The listing builds one solid part. Answer for the finished solid, in the listing's coordinates (mm). Face numbers are marked on the shaded views. A direction names the side the tool comes from. Give positions to 0.01 mm unless a question says otherwise; leave off trailing zeros. Loops run counter-clockwise (first coordinate to the right, second up) from the corner with the lowest first, then second, coordinate; pieces in that order, holes last. Notation, with made-up numbers: M -32,-33.5 L 12,-33.5 A32 cw 12,5.5 Z; hole C 39.5,84 d5. An arc over 180 degrees is marked long. One line per item, written item: value. Start each with the question number.
Q1. A cutting plane is placed at A-A, the plane x = 0. Determine the outline of the cut face in (y, z) (3 decimals), and give its area (3 significant figures).
Q2. The mould has two halves that part along Y. Classify the marked faces 1, 2 and 3: +Y half, -Y half, draft (parallel to the pull), parting line (faces both ways), or undercut.
Q3. A cutting plane is placed at C-C, the plane z = -1. Determine the outline of the cut face in (x, y) (3 decimals).
Q4. A cutting plane is placed at D-D, the plane z = 2.25. Determine the outline of the cut face in (x, y), and give its area (3 significant figures).
Q5. Flat-ended cylindrical pins translate along their axes: pin 1 (12 mm diameter, centred on x = 0, y = 0, fed in from +Z); pin 2 (1 mm diameter, centred on y = 6.5, z = -1, fed in from -X); pin 3 (4 mm diameter, centred on x = 5.5, z = 0.5, fed in from -Y). Find the tip coordinate at first contact, or state that the pin passes through.
Q6. For the marked faces 4 and 5, determine the directions among +Z, -Z, +X, -X, +Y, -Y from which every point of the face is accessible in a straight line to the end or side of a thin tool.
Q7. Consider L1, parallel to Y at x = 0, z = 1.8; L2, parallel to Z at x = 3, y = 0.25. Determine where each line is inside the solid, lowest interval first.
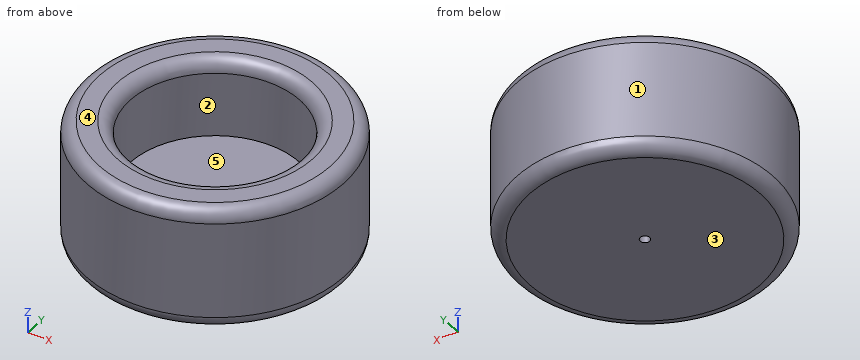
from build123d import *

# Parameters (mm, degrees)
F0_R     = 10
F1_DEPTH = 3.5
F2_R     = 10
F2_R_2   = 6.6
F3_DEPTH = 6
F4_R     = 1
F5_R     = 1
F6_R     = 0.375
F7_DEPTH = 3.501


# Not quite as in the source:
# - a feature names something its author has since deleted; it is built from what else it names


with BuildPart() as f1:
    # F0 (on Top) → F1 (new body)
    with BuildSketch(Plane.XY):
        Circle(F0_R)
    extrude(amount=-F1_DEPTH)

    # F2 (on face) → F3 (join)
    with BuildSketch(Plane.XY):
        Circle(F2_R)
        Circle(F2_R_2, mode=Mode.SUBTRACT)
    extrude(amount=F3_DEPTH)

    # F4
    f4_edges = [f1.edges().sort_by_distance(p)[0] for p in [
        (-6.6, 0, 6),
        (-10, 0, -3.5),
    ]]
    fillet(f4_edges, radius=F4_R)

    # F5
    f5_edges = [f1.edges().sort_by_distance(p)[0] for p in [
        (-10, 0, 6),
    ]]
    fillet(f5_edges, radius=F5_R)

    # F6 (on face) → F7 (cut, through all)
    with BuildSketch(Plane.XY):
        Circle(F6_R)
    extrude(amount=-F7_DEPTH, mode=Mode.SUBTRACT)


solid = f1.part
Answer block:
1. outline: M -10,-2.5 A1 ccw -9,-3.5 L -0.375,-3.5 L -0.375,0 L -6.6,0 L -6.6,5 A1 ccw -7.6,6 L -9,6 A1 ccw -10,5 Z; M 0.375,-3.5 L 9,-3.5 A1 ccw 10,-2.5 L 10,5 A1 ccw 9,6 L 7.6,6 A1 ccw 6.6,5 L 6.6,0 L 0.375,0 Z
1. area: 107 mm^2
2. face 1: parting line
2. face 2: undercut
2. face 3: draft
3. outline: C 0,0 d20; hole C 0,0 d0.75
4. outline: C 0,0 d20; hole C 0,0 d13.2
4. area: 177 mm^2
5. pin 1: z = 0
5. pin 2: x = -8
5. pin 3: y = -9.37
6. face 4: +Z, +X, -X, +Y, -Y
6. face 5: +Z
7. L1: -10 to -6.6, 6.6 to 10
7. L2: -3.5 to 0
